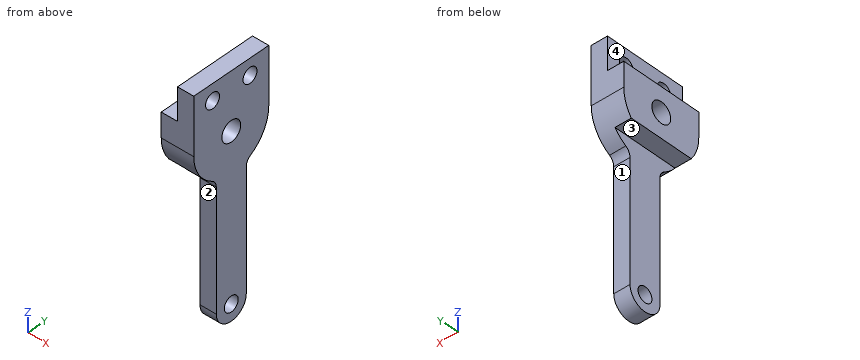
from build123d import *

# Parameters (mm, degrees)
SKETCH1_R             = 2
BOSS_EXTRUDE1_DEPTH   = 6.35
FILLET1_R             = 1.8415
SKETCH2_W             = 6.35
SKETCH2_H             = 15.875
SKETCH2_W_2           = 42.387227331
SKETCH2_H_2           = 26.263521184
CUT_EXTRUDE1_DEPTH    = 3.175
F_4_CLEARANCE_HOLE1_D = 2.9464
F_4_CLEARANCE_HOLE2_D = 2.9464


with BuildPart() as part:
    # Sketch1 → Boss-Extrude1 (new body)
    with BuildSketch(Plane(origin=(0, 0, 0), x_dir=(0, 0, -1), z_dir=(1, 0, 0))):
        with BuildLine():
            Line((-11.1125, 7.9375), (0, 7.9375))
            ThreePointArc((0, 7.9375), (4.3475478, 6.640988961), (7.274838916, 3.175))
            Line((7.274838916, 3.175), (31.75, 3.175))
            ThreePointArc((31.75, 3.175), (34.925, 0), (31.75, -3.175))
            Line((31.75, -3.175), (7.274838916, -3.175))
            ThreePointArc((7.274838916, -3.175), (4.3475478, -6.640988961), (0, -7.9375))
            Line((0, -7.9375), (-11.1125, -7.9375))
            Line((-11.1125, -7.9375), (-11.1125, 7.9375))
        make_face()
        Circle(SKETCH1_R, mode=Mode.SUBTRACT)
    extrude(amount=BOSS_EXTRUDE1_DEPTH)

    # Fillet1
    fillet1_edges = [part.edges().sort_by_distance(p)[0] for p in [
        (3.175, 3.175, -7.274838916),
        (3.175, -3.175, -7.274838916),
    ]]
    fillet(fillet1_edges, radius=FILLET1_R)

    # Sketch2 → Cut-Extrude1 (cut)
    with BuildSketch(Plane.ZY):
        with Locations((7.9375, 0)):
            Rectangle(SKETCH2_W, SKETCH2_H)
        with Locations((-25.956113666, -1.270701279)):
            Rectangle(SKETCH2_W_2, SKETCH2_H_2)
    extrude(amount=-CUT_EXTRUDE1_DEPTH, mode=Mode.SUBTRACT)

    # #4 Clearance Hole1 (through all)
    with Locations(Plane(origin=(6.35, 0, 0), x_dir=(0, 0, -1), z_dir=(1, 0, 0))):
        with Locations((-7.9375, 3.96875), (-7.9375, -3.96875)):
            Hole(F_4_CLEARANCE_HOLE1_D / 2)

    # #4 Clearance Hole2 (through all)
    with Locations(Plane.ZY.offset(-3.175)):
        with Locations((-31.75, 0)):
            Hole(F_4_CLEARANCE_HOLE2_D / 2)


solid = part.part
Work out the finished part from the listing and answer in its coordinate system (mm). Face numbers are marked on the shaded views. A direction names the side the tool comes from. Round coordinates to 2 decimals unless told otherwise and drop trailing zeros. Loops run counter-clockwise (first coordinate to the right, second up) from the corner with the lowest first, then second, coordinate; pieces in that order, holes last. Notation, with made-up numbers: (53, 39.5) -> (96, 39.5) arc R16 cw to (96, 64.5) -> close; hole circle Ø2 at (78.25, 36.5). An arc over 180 degrees is marked (long way). Use one line per item in the form item = value.
(1) A tool of negligible diameter and unlimited length cuts with its end or side. For the marked faces 1, 2, 3 and 4, from which of +Z, -Z, +X, -X, +Y, -Y can it reach the whole face along a straight path? Write none if from no direction.
Answer list:
face_1 = -Z, +X, -X, +Y
face_2 = -Z, +X, -X, -Y
face_3 = -Z, -X, +Y, -Y
face_4 = +Z, -X, +Y, -Y
(2) Straight lines are drawn through the part: line 1 (Z direction, x = 6, y = -1.25); line 2 (Z direction, x = 2, y = 2.25); line 3 (X direction, y = -0.5, z = -5) (3 decimals). For each, find the intervals that lie inside material, in ascending order.
Answer list:
line_1 = -34.67 to -32.53, -30.97 to -1.56, 1.56 to 11.11
line_2 = -4.76 to 4.76
line_3 = 3.175 to 6.35
(3) Find section A-A on y = 0. Give the number of separate pieces and of enclosed holes in the cut face, then the cut area to 3 significant figures.
Answer list:
separate_pieces = 3
enclosed_holes = 0
area = 142 mm2
(4) Find section C-C on z = -1. Give the vertices of the cut face in (x, y), then the cut area to 3 significant figures.
Answer list:
outline = (0, -7.87) -> (6.35, -7.87) -> (6.35, -1.73) -> (0, -1.73) -> close; (0, 1.73) -> (6.35, 1.73) -> (6.35, 7.87) -> (0, 7.87) -> close
area = 78.0 mm2
(5) Flat-ended cylindrical pins translate along their axes: P1, Ø4, axis at y = 2.5, z = -13, coming from the -X side (3 decimals); P2, Ø1.6, axis at x = 2, y = -2, coming from the -Z side; P3, Ø1.8, axis at y = -3.97, z = 7.94, coming from the +X side; P4, Ø3.5, axis at x = 4.5, z = -24.5, coming from the -Y side (3 decimals). Find the tip coordinate at first contact, or state that the pin passes through.
Answer list:
P1 = 3.175
P2 = -4.76
P3 = through
P4 = -3.175
